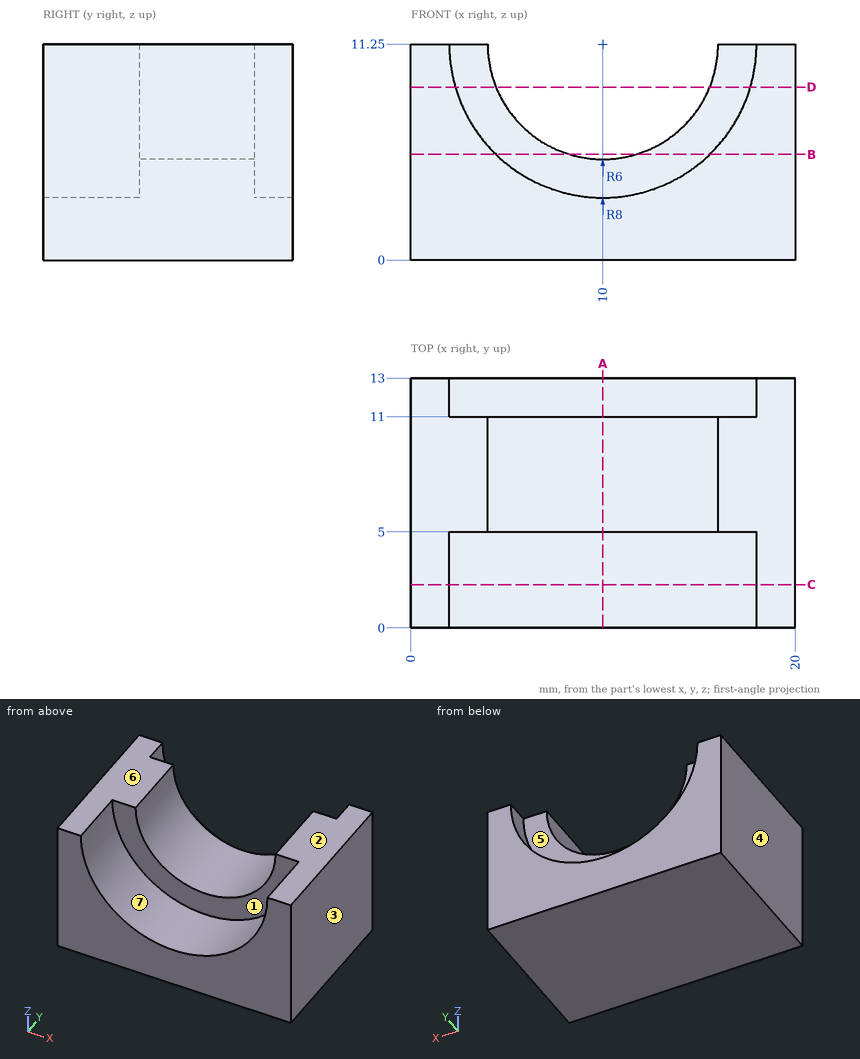
Design review of the part shown in the three views and the two pictorial views. Dimensions are in mm from the part's minimum x, y and z. A direction names the side the tool comes from. Coordinates: 2 decimals unless noted, no trailing zeros. Loops run counter-clockwise (first coordinate to the right, second up) from the corner with the lowest first, then second, coordinate; pieces in that order, holes last.
(1) Consider section B-B, the plane z = 5.5. Give the boundary of the cut face in (x, y), plus the area to 3 significant figures.
Determined:
outline: (0, 0) - (4.44, 0) - (4.44, 5) - (8.29, 5) - (8.29, 11) - (4.44, 11) - (4.44, 13) - (0, 13) - close; (11.71, 5) - (15.56, 5) - (15.56, 0) - (20, 0) - (20, 13) - (15.56, 13) - (15.56, 11) - (11.71, 11) - close
area: 162 mm2
(2) Consider section A-A, the plane x = 10. Give the boundary of the cut face in (y, z).
Determined:
outline: (0, 0) - (13, 0) - (13, 3.25) - (11, 3.25) - (11, 5.25) - (5, 5.25) - (5, 3.25) - (0, 3.25) - close
(3) Tool access review of the marked faces 5, 6 and 7: name each direction out of +Z, -Z, +X, -X, +Y, -Y from which nothing blocks a thin tool from reaching the whole face with its end or side.
Determined:
face 5: +Z, +Y
face 6: +Z, +X, -X, +Y, -Y
face 7: +Z, -Y
(4) Consider section D-D, the plane z = 9. Give the boundary of the cut face in (x, y), plus the area to 3 significant figures.
Determined:
outline: (0, 0) - (2.32, 0) - (2.32, 5) - (4.44, 5) - (4.44, 11) - (2.32, 11) - (2.32, 13) - (0, 13) - close; (15.56, 5) - (17.68, 5) - (17.68, 0) - (20, 0) - (20, 13) - (17.68, 13) - (17.68, 11) - (15.56, 11) - close
area: 85.8 mm2
(5) Wall thickness on L1, parallel to X at y = 3.5, z = 8.75; L2, parallel to X at y = 8.25, z = 6.75; L3, parallel to Y at x = 13, z = 6: over which ranges is each line inside the solid? List them lowest first.
Determined:
L1: x = 0 to 2.4, 17.6 to 20
L2: x = 0 to 6.03, 13.97 to 20
L3: y = 5 to 11
(6) Consider section C-C, the plane y = 2.25. Give the boundary of the cut face in (x, z), plus the area to 3 significant figures.
Determined:
outline: (0, 0) - (20, 0) - (20, 11.25) - (18, 11.25) arc R8 cw to (2, 11.25) - (0, 11.25) - close
area: 124 mm2
(7) Insertion check: P1, Ø6.5, axis at x = 12.5, z = 9, coming from the +Y side. The pin has a flat end and moves straight along its axis. Give the tip position at first contact, or say it passes through.
Determined:
P1: stops at y = 11
(8) Draft analysis for pull direction X (two halves, no side actions). For the marked faces 1, 2, 3 and 4, state which applies: +X half, -X half, draft (parallel to the pull), parting line (faces both ways), or undercut.
Determined:
face 1: undercut
face 2: draft
face 3: +X half
face 4: -X half
